```python
from build123d import *

# Parameters (mm, degrees)
ESQUISSE1_R         = 4
BOSS_EXTRU_1_DEPTH  = 5
ESQUISSE5_R         = 3
BOSS_EXTRU_5_DEPTH  = 5
ESQUISSE6_R         = 2.75
BOSS_EXTRU_6_DEPTH  = 5
ESQUISSE7_R         = 3
BOSS_EXTRU_7_DEPTH  = 5
ESQUISSE8_R         = 2.75
BOSS_EXTRU_8_DEPTH  = 5
ESQUISSE9_R         = 3
BOSS_EXTRU_9_DEPTH  = 5
CHANFREIN1_SIZE     = 1
ESQUISSE10_R        = 2
BOSS_EXTRU_10_DEPTH = 3
ESQUISSE11_R        = 2.5
BOSS_EXTRU_11_DEPTH = 5
CHANFREIN2_SIZE     = 1


with BuildPart() as part:
    # Esquisse1 → Boss.-Extru.1 (new body)
    with BuildSketch(Plane.XY):
        Circle(ESQUISSE1_R)
    extrude(amount=BOSS_EXTRU_1_DEPTH)

    # Esquisse5 → Boss.-Extru.5 (add)
    with BuildSketch(Plane(origin=(0, 0, 0), x_dir=(-1, 0, 0), z_dir=(0, 0, -1))):
        Circle(ESQUISSE5_R)
    extrude(amount=BOSS_EXTRU_5_DEPTH)

    # Esquisse6 → Boss.-Extru.6 (add)
    with BuildSketch(Plane(origin=(0, 0, -5), x_dir=(-1, 0, 0), z_dir=(0, 0, -1))):
        Circle(ESQUISSE6_R)
    extrude(amount=BOSS_EXTRU_6_DEPTH)

    # Esquisse7 → Boss.-Extru.7 (add)
    with BuildSketch(Plane(origin=(0, 0, -10), x_dir=(-1, 0, 0), z_dir=(0, 0, -1))):
        Circle(ESQUISSE7_R)
    extrude(amount=BOSS_EXTRU_7_DEPTH)

    # Esquisse8 → Boss.-Extru.8 (add)
    with BuildSketch(Plane(origin=(0, 0, -15), x_dir=(-1, 0, 0), z_dir=(0, 0, -1))):
        Circle(ESQUISSE8_R)
    extrude(amount=BOSS_EXTRU_8_DEPTH)

    # Esquisse9 → Boss.-Extru.9 (add)
    with BuildSketch(Plane(origin=(0, 0, -20), x_dir=(-1, 0, 0), z_dir=(0, 0, -1))):
        Circle(ESQUISSE9_R)
    extrude(amount=BOSS_EXTRU_9_DEPTH)

    # Chanfrein1
    chanfrein1_edges = [part.edges().sort_by_distance(p)[0] for p in [
        (3, 0, -25),
    ]]
    chamfer(chanfrein1_edges, length=CHANFREIN1_SIZE)

    # Esquisse10 → Boss.-Extru.10 (add)
    with BuildSketch(Plane.XY.offset(5)):
        Circle(ESQUISSE10_R)
    extrude(amount=BOSS_EXTRU_10_DEPTH)

    # Esquisse11 → Boss.-Extru.11 (add)
    with BuildSketch(Plane.XY.offset(8)):
        Circle(ESQUISSE11_R)
    extrude(amount=BOSS_EXTRU_11_DEPTH)

    # Chanfrein2
    chanfrein2_edges = [part.edges().sort_by_distance(p)[0] for p in [
        (-2.5, 0, 13),
    ]]
    chamfer(chanfrein2_edges, length=CHANFREIN2_SIZE)


solid = part.part
```
Check sheet for the modelled part. Datum: model origin and axes. Units: mm. A direction names the side the tool comes from. Round coordinates to 2 decimals unless told otherwise and drop trailing zeros. Write each loop counter-clockwise with the first axis right and the second up, starting at its lowest first coordinate (ties: lowest second). Pieces come first, ordered by that corner, then holes. Notation, with made-up numbers: M 49,17 L 82,17 A8 cw 82,30 Z; hole C 33,71 d8. An arc over 180 degrees is marked long. Write item = value, one per line. Start each with the question number.
1. Release check for a two-part mould opening along Z. For faces 1 (the flat face through (-1, 2, 8)), 2 (the cylindrical face through (-0.867, -3.905, 2.465)), 3 (the flat face through (0, 0, 13)) record: pulls with the +Z half, pulls with the -Z half, needs draft (parallel to the pull), parting line crosses it, or undercut.
2. Scan lines: line 1 (Y direction, x = 0, z = -14); line 2 (Z direction, x = 3.25, y = -0.5); line 3 (X direction, y = -2, z = -3.5). Record each from-to range of solid material in increasing order. Write a range as [from, to].
3. Section check B-B, the plane z = -10.5. Record the cut outline in (x, y), then the cut area to 3 significant figures.
4. Section check A-A, the plane z = 3. Record the cut outline in (x, y), then the cut area to 3 significant figures.
5. Gauge pin test, flat end, axial feed: pin 1 (1.5 mm diameter, centred on x = 3, z = -20.5, fed in from -Y). Record the tip position at first contact, or that the pin passes through.
6. Tool access check on faces 4 (the flat face through (1, 3, 0)), 5 (the flat face through (0, 0, -25)), 6 (the cylindrical face through (-0.54, -2.44, 9.97)), 7 (the cylindrical face through (0, -2, 6)). Record the directions out of +Z, -Z, +X, -X, +Y, -Y that give a thin tool (end or side, any length) a straight path to the whole face; none if there is none.
Results found:
q1.face_1 = undercut
q1.face_2 = needs draft
q1.face_3 = pulls with the +Z half
q2.line_1 = [-3, 3]
q2.line_2 = [0, 5]
q2.line_3 = [-2.24, 2.24]
q3.outline = C 0,0 d6
q3.area = 28.3 mm^2
q4.outline = C 0,0 d8
q4.area = 50.3 mm^2
q5.pin_1 = -1.98
q6.face_4 = -Z
q6.face_5 = -Z, +X, -X, +Y, -Y
q6.face_6 = +Z
q6.face_7 = none
